Geometry: final body of the model. Coordinates: model frame, mm. A direction names the side the tool comes from. Coordinates: 2 decimals unless noted, no trailing zeros. Loops run counter-clockwise (first coordinate to the right, second up) from the corner with the lowest first, then second, coordinate; pieces in that order, holes last. Notation, with made-up numbers: (7, 32) - (30, 32) arc R11 cw to (30, 43) - close; hole circle Ø7 at (26, 33). An arc over 180 degrees is marked (long way). Return JSON: item names as keys, results as strings.
from build123d import *

# Parameters (mm, degrees)
SALIENTE_EXTRUIR1_DEPTH = 7
CROQUIS2_R              = 27.75
SALIENTE_EXTRUIR2_DEPTH = 6
CROQUIS3_R              = 11.5
SALIENTE_EXTRUIR3_DEPTH = 6.7
NERVIO5_START           = -18.11144548
NERVIO5_OUTLINE_W       = 2.3
NERVIO5_OUTLINE_H       = 7.124259241
NERVIO5_DEPTH           = 15.309418884
MATRIZC1_COUNT          = 12
CROQUIS5_R              = 8.65
SALIENTE_EXTRUIR4_DEPTH = 3.2
CHAFL_N1_SIZE           = 2.9
CHAFL_N1_SIZE_2         = 3.2


# Read off the part's stored shape, not the designer's step: Nervio5
with BuildPart() as part:
    # Croquis1 → Saliente-Extruir1 (new body)
    with BuildSketch(Plane(origin=(0, 0, 0), x_dir=(1, 0, 0), z_dir=(0, 1, 0))):
        with BuildLine():
            Line((-7.5, -39), (7.5, -39))
            Line((7.5, -39), (7.5, -26.717269696))
            ThreePointArc((7.5, -26.717269696), (19.622213178, -19.622213178), (26.717269696, -7.5))
            Line((26.717269696, -7.5), (39, -7.5))
            Line((39, -7.5), (39, 7.5))
            Line((39, 7.5), (26.717269696, 7.5))
            ThreePointArc((26.717269696, 7.5), (19.622213178, 19.622213178), (7.5, 26.717269696))
            Line((7.5, 26.717269696), (7.5, 39))
            Line((7.5, 39), (-7.5, 39))
            Line((-7.5, 39), (-7.5, 26.717269696))
            ThreePointArc((-7.5, 26.717269696), (-19.622213178, 19.622213178), (-26.717269696, 7.5))
            Line((-26.717269696, 7.5), (-39, 7.5))
            Line((-39, 7.5), (-39, -7.5))
            Line((-39, -7.5), (-26.717269696, -7.5))
            ThreePointArc((-26.717269696, -7.5), (-19.622213178, -19.622213178), (-7.5, -26.717269696))
            Line((-7.5, -26.717269696), (-7.5, -39))
        make_face()
    extrude(amount=SALIENTE_EXTRUIR1_DEPTH)

    # Croquis2 → Saliente-Extruir2 (add)
    with BuildSketch(Plane(origin=(0, 7, 0), x_dir=(1, 0, 0), z_dir=(0, 1, 0))):
        with Locations(Location((0, 0, 0), (0, 0, 105.680350135))):
            Circle(CROQUIS2_R)
    extrude(amount=SALIENTE_EXTRUIR2_DEPTH)

    # Croquis3 → Saliente-Extruir3 (add)
    with BuildSketch(Plane(origin=(0, 13, 0), x_dir=(1, 0, 0), z_dir=(0, 1, 0))):
        with Locations(Location((0, 0, 0), (0, 0, 270))):
            Circle(CROQUIS3_R)
    extrude(amount=SALIENTE_EXTRUIR3_DEPTH)

    # Nervio5 outline → Nervio5 (add)
    with BuildSketch(Plane(origin=(0, 0, 0), x_dir=(1, 0, 0), z_dir=(0, 0.4011747826314881, 0.9160015249881293)).offset(NERVIO5_START)):
        with Locations((0, 18.562129621)):
            Rectangle(NERVIO5_OUTLINE_W, NERVIO5_OUTLINE_H)
    nervio5 = extrude(amount=NERVIO5_DEPTH)

    # MatrizC1: Nervio5 ×12 about axis
    matrizc1_axis = Axis((0, 0, 0), (0, 1, 0))
    for i in range(1, MATRIZC1_COUNT):
        add(nervio5.rotate(matrizc1_axis, i * 360 / MATRIZC1_COUNT))

    # Croquis5 → Saliente-Extruir4 (add)
    with BuildSketch(Plane(origin=(0, 19.7, 0), x_dir=(1, 0, 0), z_dir=(0, 1, 0))):
        with Locations(Location((0, 0, 0), (0, 0, 270))):
            Circle(CROQUIS5_R)
    extrude(amount=SALIENTE_EXTRUIR4_DEPTH)

    # Chaflán1
    # the kernel refuses this chamfer: 3.2, 2.9 mm, written as the material it adds along each edge
    with BuildSketch(Plane(origin=(0, 19.7, 0), x_dir=(0, 0, 1), z_dir=(-1, 0, 0))) as chafl_n1_piece_1_section:
        Polygon((8.65 + CHAFL_N1_SIZE, 0), (8.65, CHAFL_N1_SIZE_2), (8.65, 0), align=None)
    chafl_n1_piece_1 = revolve(axis=Axis((0, 19.7, 0), (0, 1, 0)), mode=Mode.PRIVATE)
    chafl_n1_piece_1 = chafl_n1_piece_1 & Plane(origin=(0, 21.282250987, 0), x_dir=(0, 0, 1), z_dir=(0, -1, 0)) * Cylinder(11.5, 47, mode=Mode.PRIVATE)
    chafl_n1_piece_1 = split(chafl_n1_piece_1, bisect_by=Plane(origin=(0, 22.9, -10.02497493), z_dir=(0, -1, 0)), keep=Keep.TOP, mode=Mode.PRIVATE)
    add(chafl_n1_piece_1)


solid = part.part
Item 1: Section query A-A, the plane y = 3.75. Return loops of the section in (x, z).
Worked out:
{"outline": "(-39, -7.5) - (-26.72, -7.5) arc R27.75 ccw to (-7.5, -26.72) - (-7.5, -39) - (7.5, -39) - (7.5, -26.72) arc R27.75 ccw to (26.72, -7.5) - (39, -7.5) - (39, 7.5) - (26.72, 7.5) arc R27.75 ccw to (7.5, 26.72) - (7.5, 39) - (-7.5, 39) - (-7.5, 26.72) arc R27.75 ccw to (-26.72, 7.5) - (-39, 7.5) - close"}
Item 2: Mould query, pull axis Z, two halves, no side actions, for faces 1 (the face through (33, 3, 7.5)), 2 (the face through (33, 7, 0)), 3 (the face through (-11.4, 16.3, -1.5)), 4 (the face through (2.64, 22.75, 8.38)). Classes: +Z half, -Z half, draft (parallel to the pull), parting line (faces both ways), or undercut.
Worked out:
{"face 1": "+Z half", "face 2": "draft", "face 3": "undercut", "face 4": "parting line"}
Item 3: Section query C-C, the plane z = 0. Return loops of the section in (x, y), and give its area (3 significant figures).
Worked out:
{"outline": "(-39, 0) - (39, 0) - (39, 7) - (27.75, 7) - (27.75, 13) - (25.47, 13) - (11.5, 19.12) - (11.5, 19.76) - (8.65, 22.9) - (-8.65, 22.9) - (-11.5, 19.76) - (-11.5, 19.12) - (-25.47, 13) - (-27.75, 13) - (-27.75, 7) - (-39, 7) - close", "area": "1,180 mm^2"}
Item 4: Section query B-B, the plane x = -24. Return loops of the section in (y, z), and give its area (3 significant figures).
Worked out:
{"outline": "(0, -13.93) - (13, -13.93) - (13, -1.15) - (13.64, -1.15) - (13.64, 1.15) - (13, 1.15) - (13, 13.93) - (0, 13.93) - close", "area": "364 mm^2"}
Item 5: Ray query, probe 1 along Y at (x, z) = (-6, -34.5); probe 2 along Z at (x, y) = (7, 16.5); probe 3 along Y at (x, z) = (15, -17.5). Return the intervals inside material, ascending. Write a range as from..to.
Worked out:
{"probe 1": "0..7", "probe 2": "-14.42..-9.82, -9.12..9.12, 9.82..14.42", "probe 3": "0..13"}
Item 6: Reachability of faces 5 (the face through (-9.046, 14.67, 13.369)), 6 (the face through (33, 3, -7.5)), 7 (the face through (-14.519, 14.67, 7.054)), 8 (the face through (7.054, 14.67, -14.519)), 9 (the face through (1.15, 15, 16)) from +Z, -Z, +X, -X, +Y, -Y: full face, straight path, thin tool, end or side. Return the list, or none.
Worked out:
{"face 5": "+Y", "face 6": "-Z, +X, +Y, -Y", "face 7": "-X, +Y", "face 8": "-Z, +Y", "face 9": "+Z, +Y"}
Item 7: Section query D-D, the plane y = 11.5. Return loops of the section in (x, z).
Worked out:
{"outline": "circle Ø55.5 at (0, 0)"}
Item 8: First-contact query: pin 1 Ø2 at (x, y) = (5.5, 11) entering from -Z; pin 2 Ø5.5 at (x, y) = (-36, 4) entering from +Z; pin 3 Ø13.5 at (x, z) = (-1.5, 31.5) entering from +Y. Flat tips, straight axial feed; report the tip coordinate or a pass-through.
Worked out:
{"pin 1": "z = -27.38", "pin 2": "z = 7.5", "pin 3": "y = 13.31"}
